from build123d import *

# Parameters (mm, degrees)
EXTRUDE_1_DEPTH = 19.5


with BuildPart() as part:
    # 草图1 → 凸台-拉伸1 (new body)
    with BuildSketch(Plane(origin=(0, 0, 0), x_dir=(1, 0, 0), z_dir=(0, 1, 0))):
        with BuildLine():
            Line((-0.240061086, 3.033784066), (-2.012384688, 3.033784066))
            ThreePointArc((-2.012384688, 3.033784066), (0, -3.640540879), (2.012384688, 3.033784066))
            Line((2.012384688, 3.033784066), (0.240061086, 3.033784066))
            Line((0.240061086, 3.033784066), (0.240061086, 3.283784066))
            Line((0.240061086, 3.283784066), (-0.240061086, 3.283784066))
            Line((-0.240061086, 3.283784066), (-0.240061086, 3.033784066))
        make_face()
        with BuildLine():
            Line((-0.829156198, 1.25), (0.829156198, 1.25))
            ThreePointArc((0.829156198, 1.25), (0, -1.5), (-0.829156198, 1.25))
        make_face(mode=Mode.SUBTRACT)
    extrude(amount=EXTRUDE_1_DEPTH)


solid = part.part
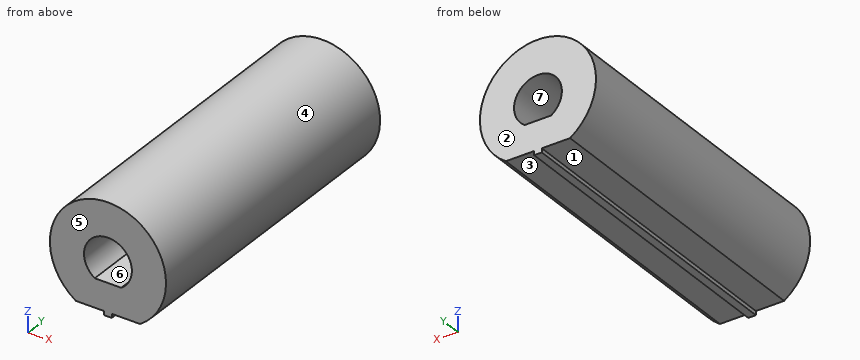
Could you check a few things on this model? Use its own coordinates, in mm. Face numbers are marked on the shaded views. A direction names the side the tool comes from. Give positions to 0.01 mm unless a question says otherwise; leave off trailing zeros. Order: outer loops, then holes, each group sorted by start corner. A loop starts at its lowest first (then second) coordinate and runs counter-clockwise, first axis right, second up. Notation, with made-up numbers: (35, 83) -> (40, 83) arc R20 ccw to (40, 119) -> close; hole circle Ø1 at (18, 50). An arc over 180 degrees is marked (long way). Answer in a Markdown table with one row per item. Add a question column.
Item 1: Imagine slicing it at B-B (x = 0). List the corners of the cut face in (y, z) for me.
Item 2: Please list where these lines run through material, in increasing order: probe 1 along X at (y, z) = (13.5, 0); probe 2 along Z at (x, y) = (0, 6.75); probe 3 along X at (y, z) = (12, -0.75).
Item 3: For the marked faces 1, 2 and 3, which set-ups out of +Z, -Z, +X, -X, +Y, -Y let a thin tool reach every point of the face, with its end or its side?
Item 4: I'm going to push flat-ended pins straight in: P1, Ø1.5, axis at y = 7.5, z = -2, coming from the -X side; P2, Ø0.5, axis at x = -1, y = 10.5, coming from the -Z side. Where does each tip first touch, or does it pass through?
Item 5: We'd pull the mould along X, two halves only. Please class the marked faces 4, 5, 6 and 7: pulls with the +X half, pulls with the -X half, needs draft (parallel to the pull), parting line crosses it, or undercut.
Item 6: Imagine slicing it at C-C (y = 11.5). List the corners of the cut face in (x, z) for me.
Item 7: Imagine slicing it at D-D (z = -1.5). List the corners of the cut face in (x, y) for me.
Item 8: Imagine slicing it at A-A (z = 0). List the corners of the cut face in (x, y) for me, and give its area (3 significant figures).
Result:
| question | item | result |
|---|---|---|
| 1 | outline | (0, -3.28) -> (19.5, -3.28) -> (19.5, -1.25) -> (0, -1.25) -> close; (0, 1.5) -> (19.5, 1.5) -> (19.5, 3.64) -> (0, 3.64) -> close |
| 2 | probe 1 | -3.64 to -1.5, 1.5 to 3.64 |
| 2 | probe 2 | -3.28 to -1.25, 1.5 to 3.64 |
| 2 | probe 3 | -3.56 to -1.3, 1.3 to 3.56 |
| 3 | face 1 | -Z, -X, +Y, -Y |
| 3 | face 2 | +Z, -Z, +X, -X, +Y |
| 3 | face 3 | -Z, +X, +Y, -Y |
| 4 | P1 | x = -3.42 |
| 4 | P2 | z = -3.03 |
| 5 | face 4 | parting line crosses it |
| 5 | face 5 | needs draft |
| 5 | face 6 | undercut |
| 5 | face 7 | undercut |
| 6 | outline | (-2.01, -3.03) -> (-0.24, -3.03) -> (-0.24, -3.28) -> (0.24, -3.28) -> (0.24, -3.03) -> (2.01, -3.03) arc R3.64 ccw (long way) to start; hole (-0.83, -1.25) -> (0.83, -1.25) arc R1.5 ccw (long way) to start |
| 7 | outline | (-3.32, 0) -> (3.32, 0) -> (3.32, 19.5) -> (-3.32, 19.5) -> close |
| 8 | outline | (-3.64, 0) -> (-1.5, 0) -> (-1.5, 19.5) -> (-3.64, 19.5) -> close; (1.5, 0) -> (3.64, 0) -> (3.64, 19.5) -> (1.5, 19.5) -> close |
| 8 | area | 83.5 mm2 |
